Read the model definition and answer for the solid it produces. Units are mm, in the model's axes. A direction names the side the tool comes from. Give positions to 0.01 mm unless a question says otherwise; leave off trailing zeros. Loops run counter-clockwise (first coordinate to the right, second up) from the corner with the lowest first, then second, coordinate; pieces in that order, holes last. Notation, with made-up numbers: (48, 36) - (52, 36) arc R20 cw to (52, 75) - close; hole circle Ø2 at (13.5, -21). An arc over 180 degrees is marked (long way). Put each result on its own line as item: value. Start each with the question number.
1. For a pull along Y with two mould halves and no side action, classify faces 4 (the flat face through (-5.784, -37.186, 44.491)), 5 (the conical face through (37.15, 11.7, 46.41)), 6 (the conical face through (34.755, 10.945, 46.236)) as released by +Y, released by -Y, zero draft, split by the parting line, or undercut.
2. For faces 1 (the flat face through (0, 0, 2.5)), 2 (the flat face through (11.732, -35, 34)), 3 (the flat face through (0, 0, 0)), determine the directions among +Z, -Z, +X, -X, +Y, -Y from which every point of the face is accessible in a straight line to the end or side of a thin tool.
3. A cutting plane is placed at A-A, the plane z = 32. Determine the outline of the cut face in (x, y), plus the area to 3 significant figures.
4. Given pin 1 Ø3 at (y, z) = (-8, 65.5) entering from +X; pin 2 Ø10 at (x, z) = (1.5, 10) entering from -Y; pin 3 Ø2 at (x, z) = (16, 32.5) entering from -Y, each flat-ended and moving along its own axis, determine where each tip first touches the part or whether it passes through.
5. Consider L1, parallel to Z at x = 6.5, y = 14.5; L2, parallel to X at y = 31.5, z = 72.5; L3, parallel to X at y = -11.5, z = 13. Determine where each line is inside the solid, lowest interval first. Write a range as from..to.
6. A cutting plane is placed at B-B, the plane x = -2. Count the separate pieces of the cut face and the enclosed holes in it, plus the area to 3 significant figures.
7. A cutting plane is placed at C-C, the plane z = 14.5. Determine the outline of the cut face in (x, y).
```python
from build123d import *

# Parameters (mm, degrees)
F0_R     = 36.5179741317
F1_DEPTH = 86
F1_TAPER = -3
F2_T     = -2.5
F4_DEPTH = 67.6
F6_DEPTH = 101
F7_R     = 3
F8_R     = 6


with BuildPart() as f1:
    # F0 (on Top) → F1 (new body)
    with BuildSketch(Plane.XY):
        Circle(F0_R)
    extrude(amount=F1_DEPTH, taper=F1_TAPER)

    # F2
    f2_openings = [f1.faces().sort_by_distance(p)[0] for p in [
        (0, 0, 86),
    ]]
    offset(amount=F2_T, openings=f2_openings, kind=Kind.INTERSECTION)

    # F3 (on Front) → F4 (cut, symmetric)
    with BuildSketch(Plane.XZ):
        Polygon((11.7323016748, 27.5090516972), (11.7323016748, 41.0563467575), (0, 47.8299942876), (-11.7323016748, 41.0563467575), (-11.7323016748, 27.5090516972), (0, 20.735404167), align=None)
    extrude(amount=F4_DEPTH, both=True, mode=Mode.SUBTRACT)

    # F5 (on Front) → F6 (cut, symmetric)
    with BuildSketch(Plane.XZ):
        with BuildLine():
            Line((29.2842475001, 110.4101017118), (-35.2238230407, 110.4101017118))
            add(Edge.make_bspline(
                [(-35.2238230407, 110.4101017118), (-29.7514190862, 103.6952824897), (-18.9586292348, 90.4497753083), (-19.7072395408, 67.0216235894), (-4.321025151, 52.1067751561), (13.9204202649, 59.2901365819), (13.1893577046, 85.3497190624), (23.5286639854, 102.6772105116), (29.2842475001, 110.4101017118)],
                knots=[0, 0, 0, 0, 0.1785016092, 0.346871767, 0.4974328306, 0.6320967895, 0.8055665743, 1, 1, 1, 1], degree=3))
        make_face()
    extrude(amount=F6_DEPTH, both=True, mode=Mode.SUBTRACT)

    # F7
    f7_edges = [f1.edges().sort_by_distance(p)[0] for p in [
        (-34.145563, 0, 2.5),
    ]]
    fillet(f7_edges, radius=F7_R)

    # F8
    f8_edges = [f1.edges().sort_by_distance(p)[0] for p in [
        (-36.517974, 0, 0),
    ]]
    fillet(f8_edges, radius=F8_R)


solid = f1.part
```
Return value:
1. face 4: zero draft
1. face 5: split by the parting line
1. face 6: undercut
2. face 1: +Z
2. face 2: +Y, -Y
2. face 3: -Z, +X, -X, +Y, -Y
3. outline: (-11.73, -36.35) - (-11.73, -33.71) arc R35.69 cw to (-11.73, 33.71) - (-11.73, 36.35) arc R38.2 ccw to start; (11.73, -36.35) arc R38.2 ccw to (11.73, 36.35) - (11.73, 33.71) arc R35.69 cw to (11.73, -33.71) - close
3. area: 462 mm2
4. pin 1: stops at x = 39.43
4. pin 2: stops at y = -37.3
4. pin 3: stops at y = -35.16
5. L1: z = 0..2.5
5. L2: x = -25.16..-20.92, 20.92..25.16
5. L3: x = -35.38..-32.73, 32.73..35.38
6. separate pieces: 3
6. enclosed holes: 0
6. area: 313 mm2
7. outline: circle Ø74.56 at (0, 0); hole circle Ø69.55 at (0, 0)
